from build123d import *

# Parameters (mm, degrees)
SKETCH_1_W          = 60
SKETCH_1_H          = 35
EXTRUDE_1_DEPTH     = 5
EXTRUDE_2_DEPTH     = 35
SKETCH_4_R          = 3
CUT_EXTRUDE_1_DEPTH = 5
SKETCH_5_R          = 1.75
CUT_EXTRUDE_2_DEPTH = 5


with BuildPart() as part:
    # Эскиз1 → Бобышка-Вытянуть1 (new body)
    with BuildSketch(Plane(origin=(0, 0, 0), x_dir=(1, 0, 0), z_dir=(0, 1, 0))):
        with Locations((30, 17.5)):
            Rectangle(SKETCH_1_W, SKETCH_1_H)
    extrude(amount=EXTRUDE_1_DEPTH)

    # Эскиз3 → Бобышка-Вытянуть2 (add)
    with BuildSketch(Plane(origin=(0, 5, 0), x_dir=(1, 0, 0), z_dir=(0, 1, 0))):
        Polygon((5, 30), (55, 30), (55, 0), (60, 0), (60, 35), (0, 35), (0, 0), (5, 0), align=None)
    extrude(amount=EXTRUDE_2_DEPTH)

    # Эскиз4 → Вырез-Вытянуть1 (cut)
    with BuildSketch(Plane(origin=(0, 0, -35), x_dir=(-1, 0, 0), z_dir=(0, 0, -1))):
        with Locations((-10, 10)):
            Circle(SKETCH_4_R)
        with Locations((-10, 30)):
            Circle(SKETCH_4_R)
        with Locations((-50, 30)):
            Circle(SKETCH_4_R)
        with Locations((-50, 10)):
            Circle(SKETCH_4_R)
    extrude(amount=-CUT_EXTRUDE_1_DEPTH, mode=Mode.SUBTRACT)

    # Эскиз5 → Вырез-Вытянуть2 (cut)
    with BuildSketch(Plane(origin=(0, 0, 0), x_dir=(-1, 0, 0), z_dir=(0, -1, 0))):
        with Locations(Location((-42, 26, 0), (0, 0, 90))):
            Circle(SKETCH_5_R)
        with Locations(Location((-18, 26, 0), (0, 0, 90))):
            Circle(SKETCH_5_R)
        with Locations(Location((-18, 4, 0), (0, 0, 90))):
            Circle(SKETCH_5_R)
        with Locations(Location((-42, 4, 0), (0, 0, 90))):
            Circle(SKETCH_5_R)
    extrude(amount=-CUT_EXTRUDE_2_DEPTH, mode=Mode.SUBTRACT)


solid = part.part
Design review of the part built by this model. Coordinates are the model's own, in mm. A direction names the side the tool comes from. Round coordinates to 2 decimals unless told otherwise and drop trailing zeros. Write each loop counter-clockwise with the first axis right and the second up, starting at its lowest first coordinate (ties: lowest second). Pieces come first, ordered by that corner, then holes. Notation, with made-up numbers: (18.5, -30) - (48.5, -30) arc R20 cw to (48.5, -2) - close; hole circle Ø11 at (42.25, 83). An arc over 180 degrees is marked (long way). Return JSON: item names as keys, results as strings. Group by question number.
Item 1: For probe 1 along X at (y, z) = (3, -4); probe 2 along Y at (x, z) = (10, -32.9); probe 3 along X at (y, z) = (9, -2), list the stretches that pass through material, from the lowest coordinate up. Write a range as [from, to].
Item 2: We need section A-A on x = 18. Write out the cut boundary in (y, z).
Item 3: We need section C-C on y = 10. Write out the cut boundary in (x, z), and give its area (3 significant figures).
Item 4: We need section B-B on z = -26. Write out the cut boundary in (x, y).
Item 5: We need section D-D on y = 22.5. Write out the cut boundary in (x, z), and give its area (3 significant figures).
Item 6: The part is to be moulded in two halves that separate along Y. For faces 1 (the face through (12.21, 32.03, -32.53)), 2 (the face through (30, 0, -18)), 3 (the face through (0, 20, -18)), say which applies: pulls with the +Y half, pulls with the -Y half, needs draft (parallel to the pull), parting line crosses it, or undercut.
Item 7: Insertion check: P1, Ø3, axis at x = 42, z = -4, coming from the +Y side; P2, Ø4.5, axis at x = 42, z = -26, coming from the +Y side; P3, Ø7, axis at x = 50, y = 10, coming from the +Z side. Each pin has a flat end and moves straight along its axis. Give the tip position at first contact, or say it passes through.
Item 8: Machinability: for faces 4 (the face through (40.29, 2.46, -25.62)), 5 (the face through (5, 22, -15)), which of the approach directions +Z, -Z, +X, -X, +Y, -Y give a long, thin tool a straight path to every point of the face, cutting with its end or side? Answer none if there is none.
Model answer:
{
 "1": {"probe 1": "x = [0, 16.25], [19.75, 40.25], [43.75, 60]", "probe 2": "y = [0, 7], [13, 27], [33, 40]", "probe 3": "x = [0, 5], [55, 60]"},
 "2": {"outline": "(0, -35) - (40, -35) - (40, -30) - (5, -30) - (5, -27.75) - (0, -27.75) - close; (0, -24.25) - (5, -24.25) - (5, -5.75) - (0, -5.75) - close; (0, -2.25) - (5, -2.25) - (5, 0) - (0, 0) - close"},
 "3": {"outline": "(0, -35) - (7, -35) - (7, -30) - (5, -30) - (5, 0) - (0, 0) - close; (13, -35) - (47, -35) - (47, -30) - (13, -30) - close; (53, -35) - (60, -35) - (60, 0) - (55, 0) - (55, -30) - (53, -30) - close", "area": "540 mm²"},
 "4": {"outline": "(0, 0) - (16.25, 0) - (16.25, 5) - (5, 5) - (5, 40) - (0, 40) - close; (19.75, 0) - (40.25, 0) - (40.25, 5) - (19.75, 5) - close; (43.75, 0) - (60, 0) - (60, 40) - (55, 40) - (55, 5) - (43.75, 5) - close"},
 "5": {"outline": "(0, -35) - (60, -35) - (60, 0) - (55, 0) - (55, -30) - (5, -30) - (5, 0) - (0, 0) - close", "area": "600 mm²"},
 "6": {"face 1": "undercut", "face 2": "pulls with the -Y half", "face 3": "needs draft"},
 "7": {"P1": "passes through", "P2": "stops at y = 5", "P3": "stops at z = -30"},
 "8": {"face 4": "+Y, -Y", "face 5": "+Z, +Y"}
}
